```python
from build123d import *

# Parameters (mm, degrees)
F0_W      = 200
F0_H      = 2.35
F0_H_2    = 14
F1_DEPTH  = 43
F4_W      = 150
F4_H      = 11.08513
F5_DEPTH  = 7
F6_R      = 1.95
F7_DEPTH  = 16.351
F9_DEPTH  = 37
F10_R     = 5
F11_R     = 0.5
F13_DEPTH = 1.55
F14_W     = 18.3
F14_H     = 3.2
F15_DEPTH = 9


with BuildPart() as f1:
    # F0 (on Top) → F1 (new body)
    with BuildSketch(Plane.XY):
        with Locations((0, 8.175)):
            Rectangle(F0_W, F0_H)
        Rectangle(F0_W, F0_H_2)
    extrude(amount=F1_DEPTH)

    # F4 (on face) → F5 (cut)
    with BuildSketch(Plane(origin=(0, 0, 0), x_dir=(1, 0, 0), z_dir=(0, 0, -1))):
        with Locations((0, 0.35)):
            Rectangle(F4_W, F4_H)
    extrude(amount=-F5_DEPTH, mode=Mode.SUBTRACT)

    # F6 (on face) → F7 (cut, through all)
    with BuildSketch(Plane.XZ.offset(7)):
        with Locations((-80, 7)):
            Circle(F6_R)
        with Locations((80, 7)):
            Circle(F6_R)
    extrude(amount=-F7_DEPTH, mode=Mode.SUBTRACT)

    # F8 (on face) → F9 (cut)
    with BuildSketch(Plane.XY.offset(43)):
        with BuildLine():
            ThreePointArc((-71.55, 3.1), (-75, -0.35), (-71.55, -3.8))
            Line((-71.55, -3.8), (71.55, -3.8))
            ThreePointArc((71.55, -3.8), (75, -0.35), (71.55, 3.1))
            Line((71.55, 3.1), (-71.55, 3.1))
        make_face()
    extrude(amount=-F9_DEPTH, mode=Mode.SUBTRACT)

    # F10
    f10_edges = [f1.edges().sort_by_distance(p)[0] for p in [
        (-100, -7, 21.5),
        (-100, 9.35, 21.5),
        (100, -7, 21.5),
        (100, 9.35, 21.5),
    ]]
    fillet(f10_edges, radius=F10_R)

    # F11
    f11_edges = [f1.edges().sort_by_distance(p)[0] for p in [
        (78.05, 9.35, 7),
        (78.05, -7, 7),
        (-81.95, -7, 7),
        (-81.95, 9.35, 7),
    ]]
    fillet(f11_edges, radius=F11_R)

    # F12 (on Front) → F13 (cut, symmetric)
    with BuildSketch(Plane.XZ):
        Polygon((-75.85, 4.603996), (-75.85, 9.396004), (-80, 11.792007), (-84.15, 9.396004), (-84.15, 4.603996), (-80, 2.207993), align=None)
        Polygon((84.15, 4.603996), (84.15, 9.396004), (80, 11.792007), (75.85, 9.396004), (75.85, 4.603996), (80, 2.207993), align=None)
    extrude(amount=F13_DEPTH, both=True, mode=Mode.SUBTRACT)

    # F14 (on face) → F15 (cut)
    with BuildSketch(Plane(origin=(0, 0, 0), x_dir=(1, 0, 0), z_dir=(0, 0, -1))):
        with Locations((-75, 0)):
            Rectangle(F14_W, F14_H)
        with Locations((75, 0)):
            Rectangle(F14_W, F14_H)
    extrude(amount=-F15_DEPTH, mode=Mode.SUBTRACT)


solid = f1.part
```
Input: part model. Units: mm. Frame: model coordinates. A direction names the side the tool comes from. Coordinates: 2 decimals unless noted, no trailing zeros. Write each loop counter-clockwise with the first axis right and the second up, starting at its lowest first coordinate (ties: lowest second). Pieces come first, ordered by that corner, then holes.
1) Material intervals for line 1 along Y through (x, z) = (31, 41); line 2 along Z through (x, y) = (80, -3.1); line 3 along X through (y, z) = (-2.25, 37), sorted ascending.
2) Section A-A on x = 51. Output: boundary loops of the cut face in (y, z), and give its area (3 significant figures).
3) Mould query, pull axis X, two halves, no side actions, for faces 4 (the flat face through (-100, 1, 21)), 5 (the flat face through (100, 1, 21)), 6 (the flat face through (-75, 3, 3)). Classes: pulls with the +X half, pulls with the -X half, needs draft (parallel to the pull), parting line crosses it, or undercut.
4) Pin query (flat end, axial travel): pin 1 Ø1 at (x, y) = (-81, -1) entering from -Z; pin 2 Ø6 at (x, y) = (-71.5, 6.5) entering from -Z; pin 3 Ø4 at (x, y) = (19.5, 3) entering from -Z. Return the tip coordinate at first contact, or that it passes through.
5) Section B-B on z = 34.5. Output: boundary loops of the cut face in (x, y), and give its area (3 significant figures).
6) Set-up query: faces 1 (the flat face through (75.3, 0.1, 9)), 2 (the cylindrical face through (75, -0.4, 25.3)), 3 (the cylindrical face through (98, -6, 22)). Return all of +Z, -Z, +X, -X, +Y, -Y with unobstructed straight access to the full face (end or side cutting, diameter ignored); none if empty.
Check result:
1. line 1: y = -7 to -3.8, 3.1 to 9.35
1. line 2: z = 0 to 5.05, 8.95 to 43
1. line 3: x = -99.99 to -74.43, 74.43 to 99.99
2. outline: (-7, 0) - (-5.89, 0) - (-5.89, 7) - (-3.8, 7) - (-3.8, 43) - (-7, 43) - close; (3.1, 7) - (5.19, 7) - (5.19, 0) - (9.35, 0) - (9.35, 43) - (3.1, 43) - close
2. area: 377 mm2
3. face 4: pulls with the -X half
3. face 5: pulls with the +X half
3. face 6: undercut
4. pin 1: stops at z = 10.93
4. pin 2: stops at z = 0
4. pin 3: stops at z = 7
5. outline: (-100, -2) arc R5 ccw to (-95, -7) - (95, -7) arc R5 ccw to (100, -2) - (100, 4.35) arc R5 ccw to (95, 9.35) - (-95, 9.35) arc R5 ccw to (-100, 4.35) - close; hole (-71.55, -3.8) - (71.55, -3.8) arc R3.45 ccw to (71.55, 3.1) - (-71.55, 3.1) arc R3.45 ccw to start
5. area: 2,220 mm2
6. face 1: -Z
6. face 2: +Z, -Z
6. face 3: +Z, -Z, +X, -Y
